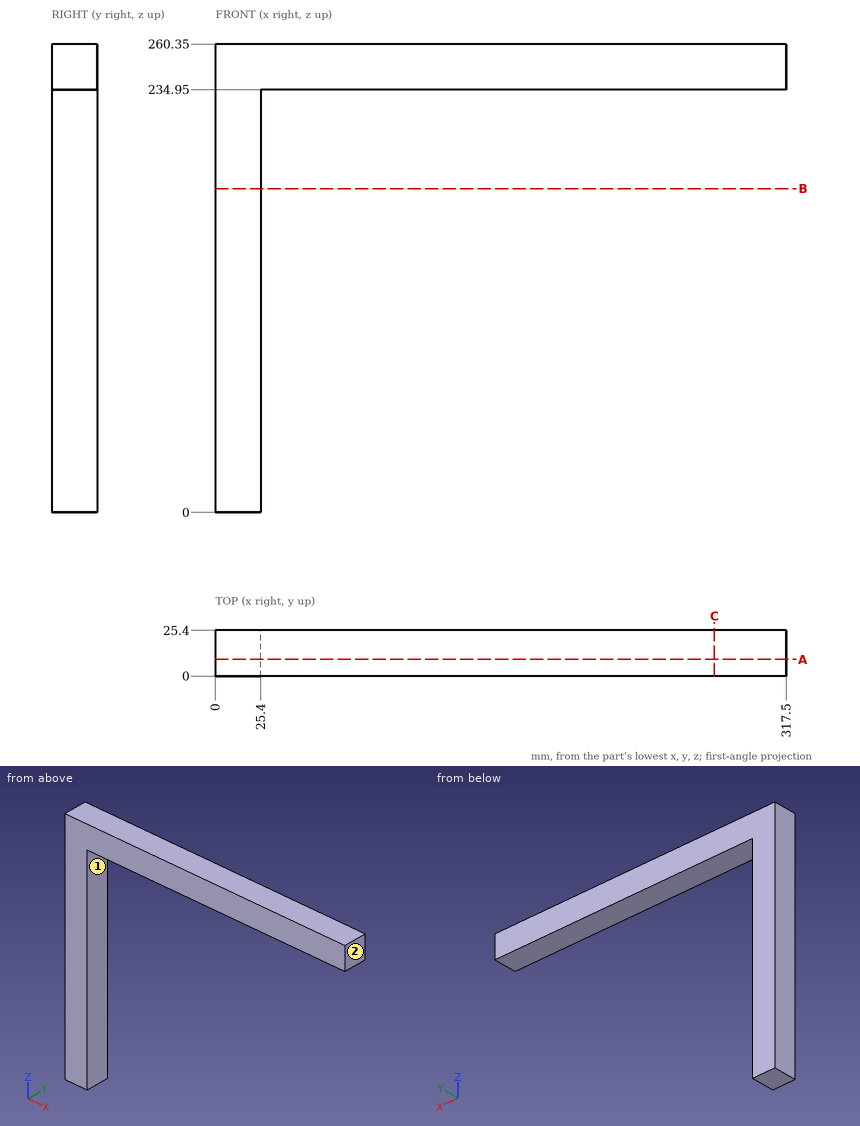
For this review, use the dimensioned drawing (mm, ordinates from the lowest corner) and the shaded views. A direction names the side the tool comes from. Round coordinates to 2 decimals unless told otherwise and drop trailing zeros. Order: outer loops, then holes, each group sorted by start corner. A loop starts at its lowest first (then second) coordinate and runs counter-clockwise, first axis right, second up. Notation, with made-up numbers: (31.5, 52) -> (37.5, 52) arc R17 cw to (37.5, 56) -> close; hole circle Ø5 at (-7.75, -14). An arc over 180 degrees is marked (long way). One line per item, written item: value. Start each with the question number.
Q1. Take a section at C-C (x = 277.5). Write out the cut boundary in (y, z), and give its area (3 significant figures).
Q2. Take a section at B-B (z = 180). Write out the cut boundary in (x, y).
Q3. Clearance check with flat-ended pins moving along their axes: pin 1 Ø1.5 at (x, y) = (69, 4.5) entering from -Z; pin 2 Ø7.5 at (y, z) = (13.5, 110) entering from +X. State where each tip first meets the part, or that it passes through.
Q4. Wall thickness on line 1 (Z direction, x = 81, y = 13.75); line 2 (X direction, y = 12.75, z = 191.5): over which ranges is each line inside the solid? List them lowest first.
Q5. Machinability: for the marked faces 1 and 2, which of the approach directions +Z, -Z, +X, -X, +Y, -Y give a long, thin tool a straight path to every point of the face, cutting with its end or side? Answer none if there is none.
Q6. Take a section at A-A (y = 9.25). Write out the cut boundary in (x, z), and give its area (3 significant figures).
Reported:
1. outline: (0, 234.95) -> (25.4, 234.95) -> (25.4, 260.35) -> (0, 260.35) -> close
1. area: 645 mm2
2. outline: (0, 0) -> (25.4, 0) -> (25.4, 25.4) -> (0, 25.4) -> close
3. pin 1: stops at z = 234.95
3. pin 2: stops at x = 25.4
4. line 1: z = 234.95 to 260.35
4. line 2: x = 0 to 25.4
5. face 1: -Z, +X, +Y, -Y
5. face 2: +Z, -Z, +X, +Y, -Y
6. outline: (0, 0) -> (25.4, 0) -> (25.4, 234.95) -> (317.5, 234.95) -> (317.5, 260.35) -> (0, 260.35) -> close
6. area: 14,000 mm2
